Autodesk Inventor part; units mm, degrees
ref_plane "YZ Plane" through (0, 0, 0) normal (1, 0, 0) x (0, 1, 0)
ref_plane "XZ Plane" through (0, 0, 0) normal (0, 1, 0) x (-1, 0, 0)
ref_plane "XY Plane" through (0, 0, 0) normal (0, 0, 1) x (1, 0, 0)
sketch "Skizze1" plane through (0, 0, 0) normal (0, 0, 1) x (1, 0, 0)
  line L0 (0, 0) -> (4.6893, 0)
  line L1 (4.6893, 0) -> (4.6893, 8.2)
  line L2 (4.6893, 8.2) -> (3.3893, 8.2)
  line L3 (3.3893, 8.2) -> (3.3893, 1.3)
  line L4 (3.3893, 1.3) -> (-4.1107, 1.3)
  line L5 (-4.1107, 1.3) -> (-4.1107, 8.2)
  line L6 (-4.1107, 8.2) -> (-5.4107, 8.2)
  line L7 (-5.4107, 8.2) -> (-5.4107, 0)
  line L8 (-5.4107, 0) -> (0, 0)
  line L9 (0, 8.5935) -> (0, -2.965) construction
  dimension "d0" = 10.1
  dimension "d2" = 8.2
  dimension "d3" = 8.2
  dimension "d4" = 1.3
  dimension "d5" = 1.3
  dimension "d6" = 1.3
extrude "Extrusion1" add sketch "Skizze1" along normal mid plane 410
sketch "Skizze2" plane through (-5.4107, 0, 205) normal (0, -1, 0) x (1, 0, 0)
  point P0 (5.4107, -205)
  point P1 (5.4107, -145)
  point P2 (5.4107, -265)
  dimension "d9" = 60
  dimension "d10" = 60
  dimension "d11" = 0
  dimension "d12" = 0
hole "Bohrung1" at (0, 0, 60) at (0, 0, -60) direction (0, 1, 0) diameter 4.3 end through all
properties part number "stab"
Model file for the job. Use its own axes, mm. A direction names the side the tool comes from. Round coordinates to 2 decimals unless told otherwise and drop trailing zeros. Order: outer loops, then holes, each group sorted by start corner. A loop starts at its lowest first (then second) coordinate and runs counter-clockwise, first axis right, second up. Notation, with made-up numbers: M -17,68 L -5,68 A17 cw -5,74 Z; hole C 17.25,48 d9. An arc over 180 degrees is marked long. Use CSV: the item, a comma, the result in double quotes.
Item 1: Probe probe 1 along Z at (x, y) = (0, 0.65); probe 2 along X at (y, z) = (6.5, 100.5); probe 3 along X at (y, z) = (0.9, 60). List the from-to ranges inside material, lowest first.
Worked answers:
probe 1,"-205 to -62.15, -57.85 to 57.85, 62.15 to 205"
probe 2,"-5.41 to -4.11, 3.39 to 4.69"
probe 3,"-5.41 to -2.15, 2.15 to 4.69"
Item 2: Pin check, flat tips, straight feed: pin 1 (1.5 mm diameter, centred on x = -0.5, z = -13, fed in from -Y); pin 2 (4 mm diameter, centred on x = -1, z = -10, fed in from +Y). Stop position of each tip, or through.
Worked answers:
pin 1,"y = 0"
pin 2,"y = 1.3"
Item 3: Saw through at B-B (x = 0). List the corners of the cut face in (y, z).
Worked answers:
outline,"M 0,-205 L 1.3,-205 L 1.3,-62.15 L 0,-62.15 Z; M 0,-57.85 L 1.3,-57.85 L 1.3,57.85 L 0,57.85 Z; M 0,62.15 L 1.3,62.15 L 1.3,205 L 0,205 Z"
Item 4: Which spindle directions (+Z, -Z, +X, -X, +Y, -Y) get a long thin tool onto all of the face, cutting with end or side? Do faces 1 (the face through (0, 0, -3)), 2 (the face through (0, 1.3, -3)). Say none if no direction does.
Worked answers:
face 1,"+Z, -Z, +X, -X, -Y"
face 2,"+Z, -Z, +Y"
Item 5: Saw through at A-A (y = 2.75). List the corners of the cut face in (x, z).
Worked answers:
outline,"M -5.41,-205 L -4.11,-205 L -4.11,205 L -5.41,205 Z; M 3.39,-205 L 4.69,-205 L 4.69,205 L 3.39,205 Z"
Item 6: Saw through at C-C (z = 87). List the corners of the cut face in (x, y), plus the area to 3 significant figures.
Worked answers:
outline,"M -5.41,0 L 4.69,0 L 4.69,8.2 L 3.39,8.2 L 3.39,1.3 L -4.11,1.3 L -4.11,8.2 L -5.41,8.2 Z"
area,"31.1 mm²"
Item 7: Pull direction X, two halves, no side cores. Call faces 3 (the face through (-4.111, 5, -3)), 4 (the face through (4.689, 4, -3)), 5 (the face through (0, 1, 205)): released by +X, released by -X, zero draft, split by the parting line, or undercut.
Worked answers:
face 3,"undercut"
face 4,"released by +X"
face 5,"zero draft"
